Geometry check sheet. Reference: drawing and pictorial views, mm from the part's lowest x, y, z. Round coordinates to 2 decimals unless told otherwise and drop trailing zeros. Loops run counter-clockwise (first coordinate to the right, second up) from the corner with the lowest first, then second, coordinate; pieces in that order, holes last. Notation, with made-up numbers: (-14.5, 76) -> (0.5, 76) arc R19 cw to (0.5, 95) -> close; hole circle Ø7 at (68.5, -1.5). An arc over 180 degrees is marked (long way). Use one line per item in the form item = value. Start each with the question number.
(1) Go/stop test with flat-tipped pins: pin 1 (0.9 mm diameter, centred on y = 1.5, z = 1.5, fed in from +X); pin 2 (0.9 mm diameter, centred on x = 93.5, z = 1.5, fed in from -Y); pin 3 (0.9 mm diameter, centred on x = 99, z = 1.5, fed in from -Y); pin 4 (10 mm diameter, centred on x = 28, y = 37.5, fed in from -Z). Record where each tip stops, or that it passes through.
(2) Sectioned sample at B-B (y = 8.5). Record the cut outline in (x, z).
(3) Sectioned sample at A-A (x = 50). Record the cut outline in (y, z), and give its area (3 significant figures).
(4) Material ranges on probe 1 along Y at (x, z) = (50, 0.75); probe 2 along Y at (x, z) = (49, 2.05) (1 decimal); probe 3 along X at (y, z) = (83, 1.2) (1 decimal), recorded low to high. Write a range as [from, to].
(5) Sectioned sample at C-C (z = 2.45). State how many separate pieces and enclosed holes the cut face has, and give its area (3 significant figures).
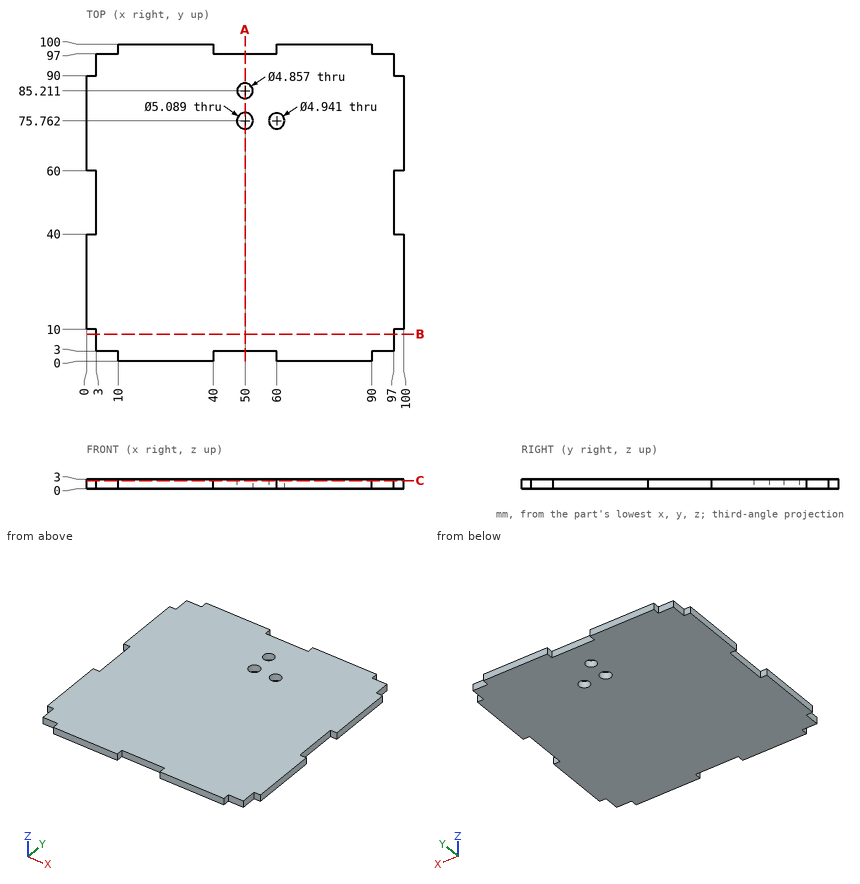
Checks:
q1.pin_1 = 90
q1.pin_2 = 3
q1.pin_3 = 10
q1.pin_4 = 0
q2.outline = (3, 0) -> (97, 0) -> (97, 3) -> (3, 3) -> close
q3.outline = (3, 0) -> (73.22, 0) -> (73.22, 3) -> (3, 3) -> close; (78.31, 0) -> (82.78, 0) -> (82.78, 3) -> (78.31, 3) -> close; (87.64, 0) -> (97, 0) -> (97, 3) -> (87.64, 3) -> close
q3.area = 252 mm2
q4.probe_1 = [3, 73.22], [78.31, 82.78], [87.64, 97]
q4.probe_2 = [3, 73.4], [78.1, 83], [87.4, 97]
q4.probe_3 = [0, 49], [51, 100]
q5.separate_pieces = 1
q5.enclosed_holes = 3
q5.area = 9,500 mm2
